Can you work these out from the model? Positions are in its coordinate system, mm. Give positions to 0.01 mm unless a question says otherwise; leave off trailing zeros. Loops run counter-clockwise (first coordinate to the right, second up) from the corner with the lowest first, then second, coordinate; pieces in that order, holes last. Notation, with made-up numbers: (43.5, 74) - (80.5, 74) arc R28 ccw to (80.5, 95) - close; hole circle Ø7 at (-14.5, -16). An arc over 180 degrees is marked (long way). Answer as a JSON object with one key per item and string values.
```python
from build123d import *

# Parameters (mm, degrees)
F1_DEPTH = 3
F2_W     = 10
F2_H     = 3
F2_H_2   = 40
F2_R     = 1.5
F3_DEPTH = 3
F5_DEPTH = 25
F7_DEPTH = 25


# Not quite as in the source:
# - a feature names something its author has since deleted; it is built from what else it names


with BuildPart() as f1:
    # F0 (on Top) → F1 (new body)
    with BuildSketch(Plane.XY):
        Polygon((25.6095033884, 1855.804875493), (-34.3904966116, 1855.804875493), (-34.3904966116, -144.195124507), (25.6095033884, -144.195124507), (25.6095033884, -164.195124507), (30.6095033884, -164.195124507), (30.6095033884, -144.195124507), (90.6095033884, -144.195124507), (90.6095033884, 1855.804875493), (30.6095033884, 1855.804875493), (30.6095033884, 1875.804875493), (25.6095033884, 1875.804875493), align=None)
    extrude(amount=F1_DEPTH)

    # F2 (on face) → F3 (join)
    with BuildSketch(Plane(origin=(0, 1855.804875493, 0), x_dir=(-1, 0, 0), z_dir=(0, 1, 0))):
        with Locations((9.3904966116, 1.5)):
            Rectangle(F2_W, F2_H)
        with Locations((9.3904966116, -20)):
            Rectangle(F2_W, F2_H_2)
        with Locations((9.3904966116, -35)):
            Circle(F2_R, mode=Mode.SUBTRACT)
    extrude(amount=F3_DEPTH)

    # F4 (on face) → F5 (join)
    with BuildSketch(Plane.XZ.offset(144.195124507)):
        with BuildLine():
            Line((30.6095033884, 3), (30.7075795998, 3))
            ThreePointArc((30.7075795998, 3), (25.1095033884, 1.5), (30.7075795998, 0))
            Line((30.7075795998, 0), (30.6095033884, 0))
            Line((30.6095033884, 0), (30.6095033884, 3))
        make_face()
        with BuildLine():
            ThreePointArc((30.7075795998, 0), (31.0072808673, 0.7235428647), (31.1095033884, 1.5))
            ThreePointArc((31.1095033884, 1.5), (31.0072808673, 2.2764571353), (30.7075795998, 3))
            Line((30.7075795998, 3), (30.6095033884, 3))
            Line((30.6095033884, 3), (30.6095033884, 0))
            Line((30.6095033884, 0), (30.7075795998, 0))
        make_face()
    extrude(amount=F5_DEPTH)

    # F6 (on face) → F7 (join)
    with BuildSketch(Plane(origin=(0, 1855.804875493, 0), x_dir=(-1, 0, 0), z_dir=(0, 1, 0))):
        with BuildLine():
            Line((-30.6095033884, 3), (-30.7075795998, 3))
            ThreePointArc((-30.7075795998, 3), (-31.1095033884, 1.5), (-30.7075795998, 0))
            Line((-30.7075795998, 0), (-30.6095033884, 0))
            Line((-30.6095033884, 0), (-30.6095033884, 3))
        make_face()
        with BuildLine():
            ThreePointArc((-30.7075795998, 0), (-27.3330462531, -1.3977774789), (-25.1095033884, 1.5))
            ThreePointArc((-25.1095033884, 1.5), (-27.3330462531, 4.3977774789), (-30.7075795998, 3))
            Line((-30.7075795998, 3), (-30.6095033884, 3))
            Line((-30.6095033884, 3), (-30.6095033884, 0))
            Line((-30.6095033884, 0), (-30.7075795998, 0))
        make_face()
    extrude(amount=F7_DEPTH)


solid = f1.part
```
1) Imagine slicing it at B-B on y = -14. Write out the boundary of the cut face in (x, z), and give its area (3 significant figures).
Check sheet entries:
{"outline": "(-34.39, 0) - (90.61, 0) - (90.61, 3) - (-34.39, 3) - close", "area": "375 mm2"}
2) I need wall thicknesses on L1, parallel to Z at x = -17, y = 775. Which ranges of the line are inside material? Lowest first, please.
Check sheet entries:
{"L1": "0 to 3"}
3) I'm going to push flat-ended pins straight in: P1, Ø1.5, axis at x = -19, z = 1.5, coming from the -Y side; P2, Ø2, axis at x = 48.5, y = 1600.5, coming from the +Z side; P3, Ø4, axis at x = -9.39, z = -35, coming from the +Y side. Where does each tip first touch, or does it pass through?
Check sheet entries:
{"P1": "y = -144.2", "P2": "z = 3", "P3": "y = 1858.8"}
4) If we mould it in two halves opening along Z, with no side actions, what happens to faces 1 (the flat face through (27, 870, 0)), 2 (the flat face through (29, 843, 3))? For each: released by +Z, released by -Z, zero draft, split by the parting line, or undercut.
Check sheet entries:
{"face 1": "released by -Z", "face 2": "released by +Z"}
5) Imagine slicing it at A-A on x = 57. Write out the boundary of the cut face in (y, z).
Check sheet entries:
{"outline": "(-144.2, 0) - (1855.8, 0) - (1855.8, 3) - (-144.2, 3) - close"}
